Build history of the part. All positions in model axes, mm. A direction names the side the tool comes from. Round coordinates to 2 decimals unless told otherwise and drop trailing zeros. Write each loop counter-clockwise with the first axis right and the second up, starting at its lowest first coordinate (ties: lowest second). Pieces come first, ordered by that corner, then holes.
from build123d import *

# Parameters (mm, degrees)
F0_W     = 101.6
F0_H     = 18.2135990537
F1_DEPTH = 127
F2_DEPTH = 127
F3_T     = -2.54
F4_W     = 15.4837965965
F4_H     = 25.2453684807
F5_DEPTH = 25.4
F6_R     = 3.5383368109
F7_DEPTH = 25.4
F8_R     = 5.08
F9_R     = 5.08


with BuildPart() as f1:
    # F0 (on Front) → F1 (new body)
    with BuildSketch(Plane.XZ):
        with Locations((0, -60.580225858)):
            Rectangle(F0_W, F0_H)
        Polygon((-50.8, -69.6870253848), (-76.2, -69.6870253848), (-50.8, -87.9006244385), align=None)
        Polygon((-76.2, 69.6870253848), (-76.2, -69.6870253848), (-50.8, -69.6870253848), (-50.8, -51.4734263312), (50.8, -51.4734263312), (50.8, -69.6870253848), (76.2, -69.6870253848), (76.2, 69.6870253848), align=None)
        Polygon((76.2, -69.6870253848), (50.8, -69.6870253848), (50.8, -87.9006244385), align=None)
        with Locations((0, -78.7938249116)):
            Rectangle(F0_W, F0_H)
    extrude(amount=F1_DEPTH)

    # F0 (on Front) → F2 (join)
    with BuildSketch(Plane.XZ):
        Polygon((76.2, -69.6870253848), (50.8, -69.6870253848), (50.8, -87.9006244385), align=None)
        Polygon((-76.2, 69.6870253848), (-76.2, -69.6870253848), (-50.8, -69.6870253848), (-50.8, -51.4734263312), (50.8, -51.4734263312), (50.8, -69.6870253848), (76.2, -69.6870253848), (76.2, 69.6870253848), align=None)
        with Locations((0, -78.7938249116)):
            Rectangle(F0_W, F0_H)
        with Locations((0, -60.580225858)):
            Rectangle(F0_W, F0_H)
        Polygon((-50.8, -69.6870253848), (-76.2, -69.6870253848), (-50.8, -87.9006244385), align=None)
    extrude(amount=F2_DEPTH)

    # F3
    f3_openings = [f1.faces().sort_by_distance(p)[0] for p in [
        (0, -63.5, 69.687025),
    ]]
    offset(amount=F3_T, openings=f3_openings)

    # F4 (on face) → F5 (cut)
    with BuildSketch(Plane(origin=(0, 0, -87.9006244385), x_dir=(1, 0, 0), z_dir=(0, 0, -1))):
        with Locations((33.6605012417, 42.3985421658)):
            Rectangle(F4_W, F4_H)
    extrude(amount=-F5_DEPTH, mode=Mode.SUBTRACT)

    # F6 (on face) → F7 (cut)
    with BuildSketch(Plane(origin=(0, 0, -87.9006244385), x_dir=(1, 0, 0), z_dir=(0, 0, -1))):
        with Locations((0, 64.9510771036)):
            Circle(F6_R)
    extrude(amount=-F7_DEPTH, mode=Mode.SUBTRACT)

    # F8
    f8_edges = [f1.edges().sort_by_distance(p)[0] for p in [
        (50.8, -63.5, -87.900624),
        (76.2, -63.5, -69.687025),
        (63.5, 0, -78.793825),
        (63.5, -127, -78.793825),
    ]]
    fillet(f8_edges, radius=F8_R)

    # F9
    f9_edges = [f1.edges().sort_by_distance(p)[0] for p in [
        (-76.2, -63.5, -69.687025),
        (-50.8, -63.5, -87.900624),
        (-63.5, 0, -78.793825),
        (-63.5, -127, -78.793825),
    ]]
    fillet(f9_edges, radius=F9_R)


solid = f1.part
1) Slice it at D-D (x = -29.5). Write the cut outline in (y, z).
Results:
outline: (-127, -87.9) - (0, -87.9) - (0, 69.69) - (-2.54, 69.69) - (-2.54, -85.36) - (-124.46, -85.36) - (-124.46, 69.69) - (-127, 69.69) - close
2) Slice it at A-A (x = 31). Write the cut outline in (y, z).
Results:
outline: (-127, -87.9) - (-55.02, -87.9) - (-55.02, -85.36) - (-124.46, -85.36) - (-124.46, 69.69) - (-127, 69.69) - close; (-29.78, -87.9) - (0, -87.9) - (0, 69.69) - (-2.54, 69.69) - (-2.54, -85.36) - (-29.78, -85.36) - close
3) Mould opens along X. For faces 1 (the flat face through (73.66, -63, 0)), 2 (the cylindrical face through (75.624, -64.376, -69.429)), 3 (the flat face through (-1, 0, -8)) say: released by +X, released by -X, zero draft, split by the parting line, or undercut.
Results:
face 1: undercut
face 2: released by +X
face 3: zero draft
4) Pin check, flat tips, straight feed: pin 1 Ø2 at (x, y) = (44, -102) entering from +Z; pin 2 Ø1.3 at (y, z) = (-44.5, -86.5) entering from +X; pin 3 Ø1.3 at (y, z) = (-38.5, -86.5) entering from -X. Stop position of each tip, or through.
Results:
pin 1: stops at z = -85.36
pin 2: stops at x = 53.66
pin 3: stops at x = -53.66
5) Slice it at C-C (z = -33.5). Write the cut outline in (x, y), plus the area to 3 significant figures.
Results:
outline: (-76.2, -127) - (76.2, -127) - (76.2, 0) - (-76.2, 0) - close; hole (-73.66, -124.46) - (73.66, -124.46) - (73.66, -2.54) - (-73.66, -2.54) - close
area: 1,390 mm2
6) Wall check: L1, parallel to Y at x = -14, z = 35; L2, parallel to X at y = -94, z = -50.5; L3, parallel to Y at x = 0, z = -86.7. Give the ranges that are in metal, low to high.
Results:
L1: y = -127 to -124.46, -2.54 to 0
L2: x = -76.2 to -73.66, 73.66 to 76.2
L3: y = -127 to -68.49, -61.41 to 0
7) Which spindle directions (+Z, -Z, +X, -X, +Y, -Y) get a long thin tool onto all of the face, cutting with end or side? Do faces 4 (the cylindrical face through (-0.767, -61.497, -86.648)), 5 (the flat face through (-61.99, -62.65, -76.75)). Say none if no direction does.
Results:
face 4: +Z, -Z
face 5: +Z
8) Slice it at B-B (y = -112). Write the cut outline in (x, z), plus the area to 3 significant figures.
Results:
outline: (-76.2, -67.08) arc R5.08 ccw to (-74.08, -71.21) - (-52.13, -86.95) arc R5.08 ccw to (-49.17, -87.9) - (49.17, -87.9) arc R5.08 ccw to (52.13, -86.95) - (74.08, -71.21) arc R5.08 ccw to (76.2, -67.08) - (76.2, 69.69) - (73.66, 69.69) - (73.66, -68.38) - (49.98, -85.36) - (-49.98, -85.36) - (-73.66, -68.38) - (-73.66, 69.69) - (-76.2, 69.69) - close
area: 1,110 mm2
